Answer from the drawing. Dimensions are ordinates in mm from the lowest x, y and z of the part. A direction names the side the tool comes from. Give positions to 0.01 mm unless a question says otherwise; leave off trailing zeros. Loops run counter-clockwise (first coordinate to the right, second up) from the corner with the lowest first, then second, coordinate; pieces in that order, holes last. Notation, with made-up numbers: (-9.75, 28.25) - (11.25, 28.25) arc R23 ccw to (11.25, 62.25) - close; hole circle Ø5 at (9.25, 32). An arc over 180 degrees is marked (long way). Write each question's results on one line, items separated by ' | '. Start each with the question number.
Q1. The part is cut by section C-C, the plane y = 10. Write down the section's boundary in (x, z).
Q2. Find the intervals of material crossed by line 1 (X direction, y = 10.2, z = 9.5) (1 decimal); line 2 (Z direction, x = 6, y = 26); line 3 (Y direction, x = 19, z = 5.5) (1 decimal), in increasing order. Write a range as from..to.
Q3. The part is cut by section D-D, the plane x = 12. Write down the section's boundary in (y, z) (1 decimal), plus the area to 3 significant figures.
Q4. The part is cut by section B-B, the plane x = 16.5. Write down the section's boundary in (y, z).
Q5. The part is cut by section A-A, the plane y = 16.5. Write down the section's boundary in (x, z), plus the area to 3 significant figures.
Q6. Determine the mould class of the marked faces 1, 2, 3 and 4 for opening direction Y: +Y half, -Y half, draft (parallel to the pull), parting line (faces both ways), or undercut.
Q7. For the marked faces 5 and 6, determine the directions among +Z, -Z, +X, -X, +Y, -Y from which every point of the face is accessible in a straight line to the end or side of a thin tool.
Q8. Given pin 1 (1.5 mm diameter, centred on x = 13.5, z = 9, fed in from +Y); pin 2 (1 mm diameter, centred on y = 9, z = 7, fed in from -X); pin 3 (1 mm diameter, centred on y = 11, z = 7.5, fed in from +X), each flat-ended and moving along its own axis, determine where each tip first touches the part or whether it passes through.
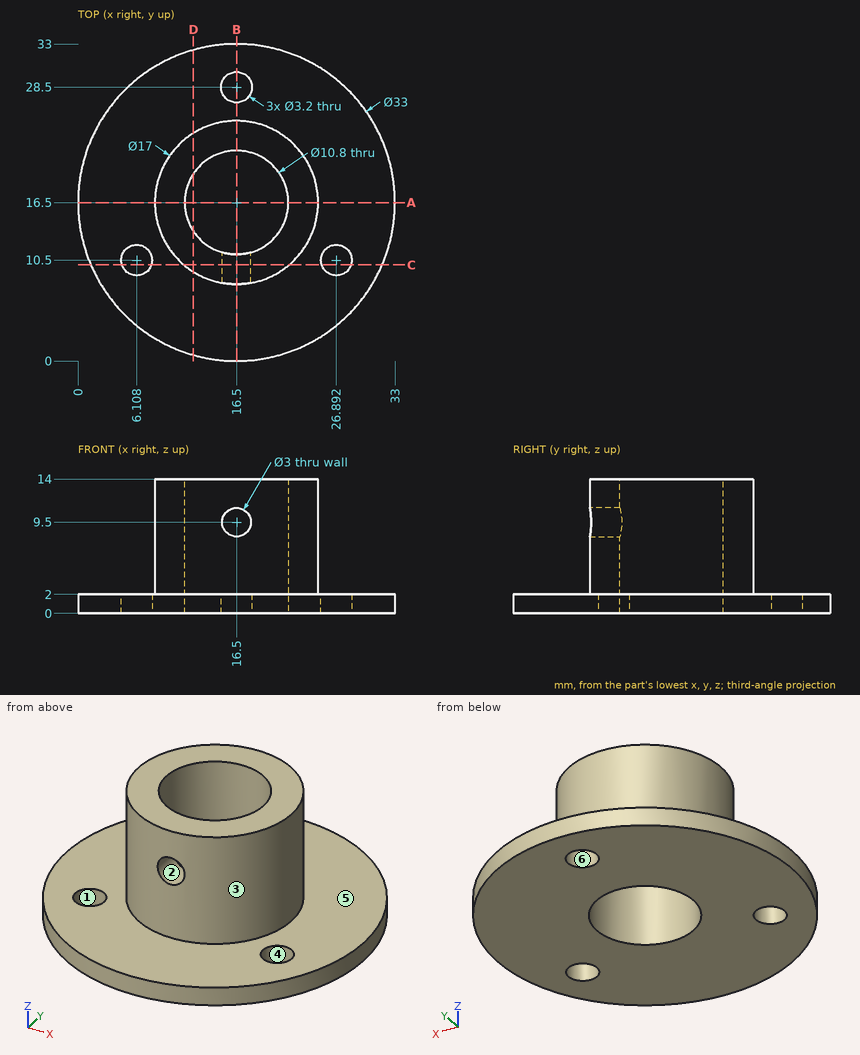
Check sheet entries:
1) outline: (1.33, 0) - (4.59, 0) - (4.59, 2) - (1.33, 2) - close; (7.63, 0) - (25.37, 0) - (25.37, 2) - (21.98, 2) - (21.98, 14) - (11.02, 14) - (11.02, 2) - (7.63, 2) - close; (28.41, 0) - (31.67, 0) - (31.67, 2) - (28.41, 2) - close; hole circle Ø3 at (16.5, 9.5)
2) line 1: x = 10.8..15, 18..22.2 | line 2: z = 0..2 | line 3: y = 8.4..11.7, 21.3..24.6
3) outline: (0.6, 0) - (13.5, 0) - (13.5, 14) - (9.3, 14) - (9.3, 2) - (0.6, 2) - close; (19.5, 0) - (32.4, 0) - (32.4, 2) - (23.7, 2) - (23.7, 14) - (19.5, 14) - close | area: 153 mm^2
4) outline: (0, 0) - (11.1, 0) - (11.1, 8) - (8, 8) - (8, 2) - (0, 2) - close; (8, 11) - (11.1, 11) - (11.1, 14) - (8, 14) - close; (21.9, 0) - (26.9, 0) - (26.9, 2) - (25, 2) - (25, 14) - (21.9, 14) - close; (30.1, 0) - (33, 0) - (33, 2) - (30.1, 2) - close
5) outline: (0, 0) - (11.1, 0) - (11.1, 14) - (8, 14) - (8, 2) - (0, 2) - close; (21.9, 0) - (33, 0) - (33, 2) - (25, 2) - (25, 14) - (21.9, 14) - close | area: 119 mm^2
6) face 1: undercut | face 2: draft | face 3: parting line | face 4: undercut
7) face 5: +Z | face 6: +Z, -Z
8) pin 1: stops at y = 24.7 | pin 2: stops at x = 11.68 | pin 3: stops at x = 23.37
